For this review, take the finished solid that the model builds, in its own axes (mm). Face numbers are marked on the shaded views. A direction names the side the tool comes from. Round coordinates to 2 decimals unless told otherwise and drop trailing zeros. Order: outer loops, then holes, each group sorted by start corner. A loop starts at its lowest first (then second) coordinate and runs counter-clockwise, first axis right, second up. Notation, with made-up numbers: (79.25, -37) - (93.25, -37) arc R17 ccw to (93.25, -21) - close; hole circle Ø6 at (6, 70.25). An arc over 180 degrees is marked (long way). One line per item, written item: value.
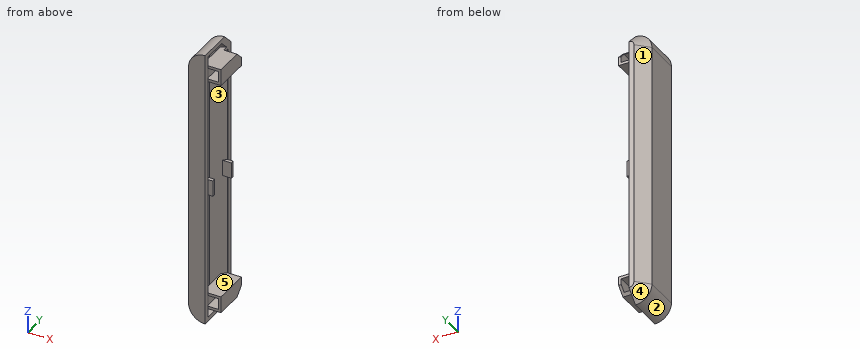
```python
from build123d import *

# Parameters (mm, degrees)
BOSS_EXTRUDE1_DEPTH      = 28
SHELL1_T                 = -2.5
SHELL1_THICKNESS_2_DEPTH = 0.5
SHELL1_THICKNESS_3_DEPTH = 0.5
CHAMFER1_SIZE            = 7
BOSS_EXTRUDE2_REACH      = 164.25
SKETCH6_W                = 11.122019094
SKETCH6_H                = 10
SKETCH6_W_2              = 6.8
SKETCH6_H_2              = 6.8
CHAMFER2_SIZE            = 3
CUT_EXTRUDE2_START       = -8
CUT_EXTRUDE2_DEPTH       = 8
BOSS_EXTRUDE3_DEPTH      = 3
BOSS_EXTRUDE3_DEPTH_BACK = 3
SKETCH8_W                = 9.684827103
SKETCH8_H                = 2


with BuildPart() as part:
    # Sketch3 → Boss-Extrude1 (new body)
    with BuildSketch(Plane(origin=(0, 0, 0), x_dir=(1, 0, 0), z_dir=(0, 1, 0))):
        with BuildLine():
            Line((0, 160), (0, -10))
            ThreePointArc((0, -10), (-7.071067812, -7.071067812), (-10, 0))
            Line((-10, 0), (-10, 150))
            ThreePointArc((-10, 150), (-7.071067812, 157.071067812), (0, 160))
        make_face()
    extrude(amount=BOSS_EXTRUDE1_DEPTH)

    # Shell1
    shell1_openings = [part.faces().sort_by_distance(p)[0] for p in [
        (0, 14, -75),
    ]]
    offset(amount=SHELL1_T, openings=shell1_openings, kind=Kind.INTERSECTION)

    # Shell1 thickness 2 face (on inner face of the shell) → Shell1 thickness 2 (add)
    with BuildSketch(Plane(origin=(-3.708717972, 2.5, -75), x_dir=(0, 0, -1), z_dir=(0, -1, 0))):
        with BuildLine():
            Line((-82.5, 3.708717972), (82.5, 3.708717972))
            ThreePointArc((82.5, 3.708717972), (80.303300859, -1.594582887), (75, -3.791282028))
            Line((75, -3.791282028), (-75, -3.791282028))
            ThreePointArc((-75, -3.791282028), (-80.303300859, -1.594582887), (-82.5, 3.708717972))
        make_face()
    extrude(amount=-SHELL1_THICKNESS_2_DEPTH)

    # Shell1 thickness 3 face (on inner face of the shell) → Shell1 thickness 3 (add)
    with BuildSketch(Plane(origin=(-3.708717972, 25.5, -75), x_dir=(0, 0, 1), z_dir=(0, 1, 0))):
        with BuildLine():
            Line((-82.5, 3.708717972), (82.5, 3.708717972))
            ThreePointArc((82.5, 3.708717972), (80.303300859, -1.594582887), (75, -3.791282028))
            Line((75, -3.791282028), (-75, -3.791282028))
            ThreePointArc((-75, -3.791282028), (-80.303300859, -1.594582887), (-82.5, 3.708717972))
        make_face()
    extrude(amount=-SHELL1_THICKNESS_3_DEPTH)

    # Chamfer1
    chamfer1_edges = [part.edges().sort_by_distance(p)[0] for p in [
        (-7.071067812, 28, 7.071067812),
        (-5.303300859, 25, -155.303300859),
        (-7.5, 25, -75),
        (-5.303300859, 25, 5.303300859),
        (-7.071067812, 28, -157.071067812),
        (-10, 28, -75),
    ]]
    chamfer(chamfer1_edges, length=CHAMFER1_SIZE)

    # Boss-Extrude2: up to this face of the body (flat: up to its plane)
    boss_extrude2_end = Plane(part.part.faces().sort_by_distance((-0.249803145, 25, -75))[0])
    # Sketch6 → Boss-Extrude2 (add, up to the picked face)
    with BuildSketch(Plane(origin=(0, 3, 0), x_dir=(1, 0, 0), z_dir=(0, 1, 0)), mode=Mode.PRIVATE) as boss_extrude2_sk1:
        with Locations((2.438990453, 147)):
            Rectangle(SKETCH6_W, SKETCH6_H)
        with Locations((3, 147)):
            Rectangle(SKETCH6_W_2, SKETCH6_H_2, mode=Mode.SUBTRACT)
    boss_extrude2_tool1 = split(extrude(boss_extrude2_sk1.sketch, amount=BOSS_EXTRUDE2_REACH, mode=Mode.PRIVATE), bisect_by=boss_extrude2_end, keep=Keep.BOTH, mode=Mode.PRIVATE)
    # Sketch6 → Boss-Extrude2 (add, up to the picked face)
    with BuildSketch(Plane(origin=(0, 3, 0), x_dir=(1, 0, 0), z_dir=(0, 1, 0)), mode=Mode.PRIVATE) as boss_extrude2_sk2:
        with Locations((2.438990453, 3)):
            Rectangle(SKETCH6_W, SKETCH6_H)
        with Locations((3, 3)):
            Rectangle(SKETCH6_W_2, SKETCH6_H_2, mode=Mode.SUBTRACT)
    boss_extrude2_tool2 = split(extrude(boss_extrude2_sk2.sketch, amount=BOSS_EXTRUDE2_REACH, mode=Mode.PRIVATE), bisect_by=boss_extrude2_end, keep=Keep.BOTH, mode=Mode.PRIVATE)
    add(boss_extrude2_tool1.solids().sort_by(Axis((2.43899, 3, -151.850434), (0, 1, 0)))[0])
    add(boss_extrude2_tool2.solids().sort_by(Axis((-2.972453, 3, -3), (0, 1, 0)))[0])

    # Chamfer2
    chamfer2_edges = [part.edges().sort_by_distance(p)[0] for p in [
        (-3.122019094, 3, -3),
        (-3.122019094, 3, -147),
    ]]
    chamfer(chamfer2_edges, length=CHAMFER2_SIZE)

    # Sketch7 → Cut-Extrude2 (cut)
    with BuildSketch(Plane(origin=(8, 0, 0), x_dir=(0, 0, -1), z_dir=(1, 0, 0)).offset(CUT_EXTRUDE2_START)):
        Polygon((-3.29028529, 29.773150155), (-3.29028529, 18.960661134), (4.456137204, 26.707083629), align=None)
        Polygon((145.543862796, 26.707083629), (153.29028529, 29.773150155), (153.29028529, 18.960661134), align=None)
    extrude(amount=CUT_EXTRUDE2_DEPTH, mode=Mode.SUBTRACT)

    # Sketch8 → Boss-Extrude3 (add, two sides: drawn at the far end of the back side and taken through both)
    with BuildSketch(Plane(origin=(0, 0, 0), x_dir=(0, 0, -1), z_dir=(1, 0, 0)).offset(-BOSS_EXTRUDE3_DEPTH_BACK)):
        with Locations((74.990759453, 4)):
            Rectangle(SKETCH8_W, SKETCH8_H)
        with Locations((74.990759453, 24)):
            Rectangle(SKETCH8_W, SKETCH8_H)
    extrude(amount=BOSS_EXTRUDE3_DEPTH + BOSS_EXTRUDE3_DEPTH_BACK)


solid = part.part
```
Item 1: Take a section at B-B (y = 13). Write out the cut boundary in (x, z), plus the area to 3 significant figures.
Returned:
outline: (-10, -150) arc R10 ccw to (0, -160) - (0, -157.5) arc R7.5 cw to (-7.5, -150) - (-7.5, 0) arc R7.5 cw to (0, 7.5) - (0, 10) arc R10 ccw to (-10, 0) - close; (-3.12, -152) - (8, -152) - (8, -142) - (-3.12, -142) - close; (-3.12, -8) - (8, -8) - (8, 2) - (-3.12, 2) - close; hole (-0.4, -150.4) - (6.4, -150.4) - (6.4, -143.6) - (-0.4, -143.6) - close; hole (-0.4, -6.4) - (6.4, -6.4) - (6.4, 0.4) - (-0.4, 0.4) - close
area: 574 mm^2
Item 2: The part is to be moulded in two halves that separate along Y. For the marked faces 1, 2 and 3, say which applies: +Y half, -Y half, draft (parallel to the pull), parting line (faces both ways), or undercut.
Returned:
face 1: +Y half
face 2: draft
face 3: undercut
Item 3: Machinability: for the marked faces 4 and 5, which of the approach directions +Z, -Z, +X, -X, +Y, -Y give a long, thin tool a straight path to every point of the face, cutting with its end or side? Answer none if there is none.
Returned:
face 4: -Z, -X, +Y
face 5: +X
Item 4: Wall thickness on line 1 (Z direction, x = 3.25, y = 15.75); line 2 (Z direction, x = -2, y = 12); line 3 (Y direction, x = -0.5, z = -100): over which ranges is each line inside the solid? List them lowest first.
Returned:
line 1: -152 to -150.4, -143.6 to -142, -8 to -6.4, 0.4 to 2
line 2: -159.8 to -157.23, -152 to -142, -8 to 2, 7.23 to 9.8
line 3: 0 to 3, 25 to 28
Item 5: Take a section at A-A (z = -145). Write out the cut boundary in (x, y), plus the area to 3 significant figures.
Returned:
outline: (-10, 0) - (0, 0) - (0, 3) - (-0.4, 3) - (-0.4, 25) - (0, 25) - (0, 28) - (-3, 28) - (-10, 21) - close; (6.4, 3) - (8, 3) - (8, 25) - (6.4, 25) - close; hole (-7.5, 3) - (-6.12, 3) - (-3.12, 6) - (-3.12, 22.38) - (-7.5, 18) - close
area: 211 mm^2
Item 6: Take a section at C-C (z = -93). Write out the cut boundary in (x, y), plus the area to 3 significant figures.
Returned:
outline: (-10, 0) - (0, 0) - (0, 3) - (-7.5, 3) - (-7.5, 18) - (-0.5, 25) - (0, 25) - (0, 28) - (-3, 28) - (-10, 21) - close
area: 115 mm^2
Item 7: For P1, Ø1, axis at x = 0, y = 23.5, coming from the -Z side; P2, Ø6, axis at x = 5.5, z = -4, coming from the +Y side; P3, Ø4, axis at x = 4.5, y = 8, coming from the -Z side; P4, Ø2, axis at x = 2, z = -27.5, coming from the +Y side, all flat-tipped, find the tip position at first contact; note any pin that passes through.
Returned:
P1: z = -158
P2: y = 25
P3: z = -152
P4: through
